The model under review builds one solid part; all positions refer to its coordinate system, in mm. Coordinates: 2 decimals unless noted, no trailing zeros. Write each loop counter-clockwise with the first axis right and the second up, starting at its lowest first coordinate (ties: lowest second). Pieces come first, ordered by that corner, then holes. Notation, with made-up numbers: M 9.25,-2.75 L 19.25,-2.75 A19 ccw 19.25,29.25 Z; hole C -10.5,22 d11. An arc over 180 degrees is marked long. Answer as a JSON object with one key per item and string values.
```python
from build123d import *

# Parameters (mm, degrees)
F0_W     = 88.9
F0_H     = 762
F1_DEPTH = 38.1
F2_W     = 914.4
F2_H     = 38.1
F3_DEPTH = 38.1
F4_W     = 88.9
F4_H     = 762
F5_DEPTH = 38.1
F6_W     = 914.4
F6_H     = 38.1
F7_DEPTH = 38.1


with BuildPart() as f1:
    # F0 (on Front) → F1 (new body)
    with BuildSketch(Plane.XZ):
        Rectangle(F0_W, F0_H)
    extrude(amount=F1_DEPTH)

    # F2 (on Front) → F3 (join)
    with BuildSketch(Plane.XZ):
        with Locations((412.75, 400.05)):
            Rectangle(F2_W, F2_H)
    extrude(amount=F3_DEPTH)

    # F4 (on Front) → F5 (join)
    with BuildSketch(Plane.XZ):
        with Locations((825.5, 0)):
            Rectangle(F4_W, F4_H)
    extrude(amount=F5_DEPTH)

    # F6 (on Front) → F7 (join)
    with BuildSketch(Plane.XZ):
        with Locations((412.75, -400.05)):
            Rectangle(F6_W, F6_H)
    extrude(amount=F7_DEPTH)


solid = f1.part
```
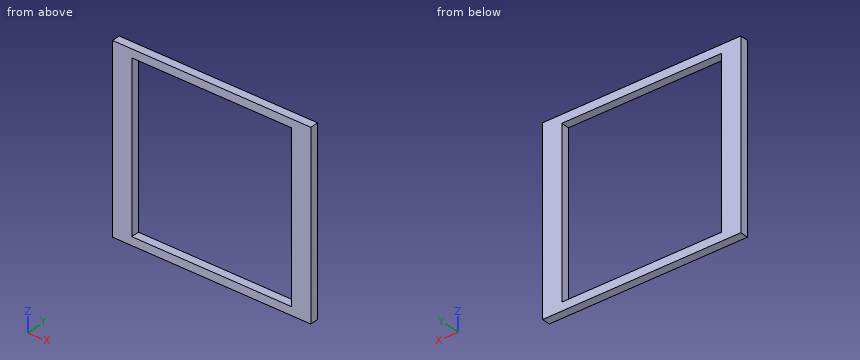
(1) Wall thickness on line 1 along X through (y, z) = (-31, 315); line 2 along Z through (x, y) = (764, -21.5): over which ranges is each line inside the solid? List them lowest first. Write a range as from..to.
Results list:
{"line 1": "-44.45..44.45, 781.05..869.95", "line 2": "-419.1..-381, 381..419.1"}
(2) Add section A-A on y = -20. Give the boundary of the cut face in (x, z).
Results list:
{"outline": "M -44.45,-419.1 L 869.95,-419.1 L 869.95,419.1 L -44.45,419.1 Z; hole M 44.45,-381 L 781.05,-381 L 781.05,381 L 44.45,381 Z"}
(3) Add section B-B on x = 682. Give the boundary of the cut face in (y, z), and give its area (3 significant figures).
Results list:
{"outline": "M -38.1,-419.1 L 0,-419.1 L 0,-381 L -38.1,-381 Z; M -38.1,381 L 0,381 L 0,419.1 L -38.1,419.1 Z", "area": "2,900 mm²"}
(4) Add section C-C on z = -151.5. Give the boundary of the cut face in (x, y), and give its area (3 significant figures).
Results list:
{"outline": "M -44.45,-38.1 L 44.45,-38.1 L 44.45,0 L -44.45,0 Z; M 781.05,-38.1 L 869.95,-38.1 L 869.95,0 L 781.05,0 Z", "area": "6,770 mm²"}
